Design review of the part built by this model. Coordinates are the model's own, in mm. Give positions to 0.01 mm unless a question says otherwise; leave off trailing zeros. Write each loop counter-clockwise with the first axis right and the second up, starting at its lowest first coordinate (ties: lowest second). Pieces come first, ordered by that corner, then holes. Notation, with made-up numbers: M -27,18 L -14,18 A33 ccw -14,55 Z; hole C -38.75,-29 d2. An arc over 180 degrees is marked long. Answer in a Markdown table with one row per item.
```python
from build123d import *

# Parameters (mm, degrees)
F0_W      = 32.1
F0_H      = 25.2
F0_W_2    = 5.4
F0_H_2    = 5.4
F1_DEPTH  = 200
F3_W      = 32.1
F3_H      = 25.2
F4_DEPTH  = 3
F5_R      = 2
F6_R      = 1.75
F7_R      = 1.75
F8_DEPTH  = 1
F9_R      = 0.99999
F10_R     = 1.75
F11_DEPTH = 1
F12_R     = 0.99999


# Not quite as in the source:
# - a fillet or chamfer is up to 0.001 mm smaller than in the source, because OpenCascade refuses the exact size


with BuildPart() as f1:
    # F0 (on Front) → F1 (new body)
    with BuildSketch(Plane.XZ):
        with Locations((-0.710526225, -0.3999928176)):
            Rectangle(F0_W, F0_H)
        Polygon((-13.760526225, -6.9499006331), (-13.760526225, -4.5999928176), (-8.360526225, -4.5999928176), (-8.360526225, -9.9999928176), (-13.760526225, -9.9999928176), align=None, mode=Mode.SUBTRACT)
        with Locations((-4.160526225, -7.2999928176)):
            Rectangle(F0_W_2, F0_H_2, mode=Mode.SUBTRACT)
        Polygon((-13.760526225, -3.0999928176), (-13.760526225, 0.7499149978), (-13.760526225, 2.3000071824), (-8.360526225, 2.3000071824), (-8.360526225, -3.0999928176), align=None, mode=Mode.SUBTRACT)
        with Locations((-4.160526225, -0.3999928176)):
            Rectangle(F0_W_2, F0_H_2, mode=Mode.SUBTRACT)
        with Locations((2.739473775, -7.2999928176)):
            Rectangle(F0_W_2, F0_H_2, mode=Mode.SUBTRACT)
        with Locations((9.639473775, -7.2999928176)):
            Rectangle(F0_W_2, F0_H_2, mode=Mode.SUBTRACT)
        with Locations((2.739473775, -0.3999928176)):
            Rectangle(F0_W_2, F0_H_2, mode=Mode.SUBTRACT)
        with Locations((9.639473775, -0.3999928176)):
            Rectangle(F0_W_2, F0_H_2, mode=Mode.SUBTRACT)
        with Locations((-11.060526225, 6.5000071824)):
            Rectangle(F0_W_2, F0_H_2, mode=Mode.SUBTRACT)
        with Locations((-4.160526225, 6.5000071824)):
            Rectangle(F0_W_2, F0_H_2, mode=Mode.SUBTRACT)
        with Locations((2.739473775, 6.5000071824)):
            Rectangle(F0_W_2, F0_H_2, mode=Mode.SUBTRACT)
        with Locations((9.639473775, 6.5000071824)):
            Rectangle(F0_W_2, F0_H_2, mode=Mode.SUBTRACT)
    extrude(amount=F1_DEPTH)

    # F3 (on face) → F4 (join)
    with BuildSketch(Plane.XZ.offset(200)):
        with Locations((-0.710526225, -0.3999928176)):
            Rectangle(F3_W, F3_H)
    extrude(amount=F4_DEPTH)

    # F5
    f5_edges = [f1.edges().sort_by_distance(p)[0] for p in [
        (15.339474, -203, -0.399993),
        (-0.710526, -203, 12.200007),
        (-16.760526, -203, -0.399993),
        (-0.710526, -203, -12.999993),
    ]]
    fillet(f5_edges, radius=F5_R)

    # F6
    f6_edges = [f1.edges().sort_by_distance(p)[0] for p in [
        (-0.710526, 0, 12.200007),
        (15.339474, 0, -0.399993),
        (-0.710526, 0, -12.999993),
        (-16.760526, 0, -0.399993),
    ]]
    fillet(f6_edges, radius=F6_R)

    # F7 (on face) → F8 (join)
    with BuildSketch(Plane.XY.offset(12.2000071824)):
        with Locations((-0.710526225, -26.75)):
            Circle(F7_R)
    extrude(amount=F8_DEPTH)

    # F9 (radius 1 in the source; OpenCascade refuses exactly that, so slightly less here)
    f9_edges = [f1.edges().sort_by_distance(p)[0] for p in [
        (-2.460526, -26.75, 13.200007),
    ]]
    fillet(f9_edges, radius=F9_R)

    # F10 (on face) → F11 (join)
    with BuildSketch(Plane(origin=(0, 0, -12.9999928176), x_dir=(1, 0, 0), z_dir=(0, 0, -1))):
        with Locations((-0.710526225, 26.75)):
            Circle(F10_R)
    extrude(amount=F11_DEPTH)

    # F12 (radius 1 in the source; OpenCascade refuses exactly that, so slightly less here)
    f12_edges = [f1.edges().sort_by_distance(p)[0] for p in [
        (-2.460526, -26.75, -13.999993),
    ]]
    fillet(f12_edges, radius=F12_R)


solid = f1.part
```
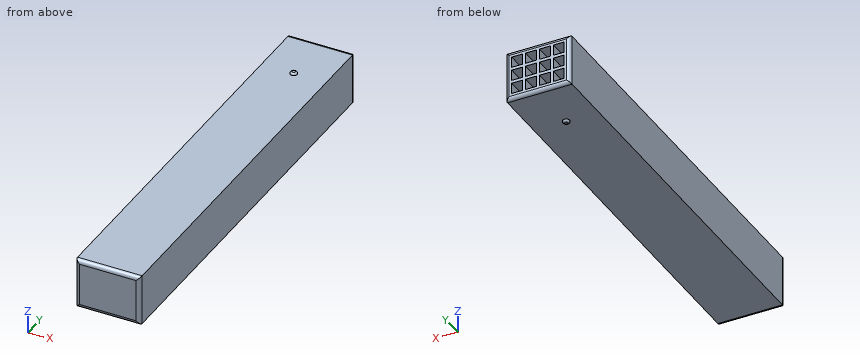
1) Add section A-A (x = 9.5). Write out the cut boundary in (y, z), and give its area (3 significant figures).
Geometry says:
| item | result |
|---|---|
| outline | M -203,-11 A2 ccw -201,-13 L -1.75,-13 A1.75 ccw 0,-11.25 L 0,-10 L -200,-10 L -200,-4.6 L 0,-4.6 L 0,-3.1 L -200,-3.1 L -200,2.3 L 0,2.3 L 0,3.8 L -200,3.8 L -200,9.2 L 0,9.2 L 0,10.45 A1.75 ccw -1.75,12.2 L -201,12.2 A2 ccw -203,10.2 Z |
| area | 1,870 mm^2 |
2) To check wall thickness, follow probe 1 along X at (y, z) = (-95, 7.75); probe 2 along Z at (x, y) = (-6.5, -99.5); probe 3 along Y at (x, z) = (5, -5.5). State the ranges of each line that lie inside material, in increasing order. Write a range as [from, to].
Geometry says:
| item | result |
|---|---|
| probe 1 | [-16.76, -13.76], [-8.36, -6.86], [-1.46, 0.04], [5.44, 6.94], [12.34, 15.34] |
| probe 2 | [-13, -10], [-4.6, -3.1], [2.3, 3.8], [9.2, 12.2] |
| probe 3 | [-203, -200] |
3) Insertion check: P1, Ø2.5, axis at x = 9, z = -8, coming from the +Y side; P2, Ø6, axis at x = -10, y = -66, coming from the +Z side; P3, Ø12, axis at x = 9, y = -130.5, coming from the -Z side. Each pin has a flat end and moves straight along its axis. Give the tip position at first contact, or say it passes through.
Geometry says:
| item | result |
|---|---|
| P1 | y = -200 |
| P2 | z = 12.2 |
| P3 | z = -13 |
4) Add section B-B (y = -109.5). Count the separate pieces of the cut face and the enclosed holes in it, and give its area (3 significant figures).
Geometry says:
| item | result |
|---|---|
| separate pieces | 1 |
| enclosed holes | 12 |
| area | 459 mm^2 |
